from build123d import *

# Parameters (mm, degrees)
BOSS_EXTRUDE5_DEPTH      = 20
BOSS_EXTRUDE5_DEPTH_BACK = 20
SKETCH6_R                = 2.6000000000000005
SKETCH7_W                = 30.000000000000004
SKETCH7_H                = 21
CUT_EXTRUDE1_DEPTH       = 16
BOSS_EXTRUDE6_DEPTH      = 18
BOSS_EXTRUDE7_DEPTH      = 4
SKETCH12_W               = 4.9999999999999964
SKETCH12_H               = 12.999999999999998
BOSS_EXTRUDE8_DEPTH      = 34
FILLET4_R                = 5
FILLET5_R                = 1
CUT_EXTRUDE3_START       = -15
CUT_EXTRUDE3_DEPTH       = 10
CUT_EXTRUDE4_DEPTH       = 3.923095079
FILLET7_R                = 5
FILLET8_R                = 50


with BuildPart() as part:
    # Sketch6 → Boss-Extrude5 (new, two sides: drawn at the far end of the back side and taken through both)
    with BuildSketch(Plane(origin=(0, 0, 0), x_dir=(0, 0, -1), z_dir=(1, 0, 0)).offset(-BOSS_EXTRUDE5_DEPTH_BACK)):
        with BuildLine():
            Line((-23, -8), (0, -8))
            ThreePointArc((0, -8), (8, 0), (0, 8))
            Line((0, 8), (-13, 7.999999999999998))
            Line((-13, 7.999999999999998), (-13, 42))
            Line((-13, 42), (-8.56466921236316, 42))
            Line((-8.56466921236316, 42), (6.542901083469773, 68.16707933130117))
            Line((6.542901083469773, 68.16707933130117), (-5.004104300322731, 68.16707933130117))
            Line((-5.004104300322731, 68.16707933130117), (-20.111674596155662, 42))
            Line((-20.111674596155662, 42), (-23, 42))
            Line((-23, 42), (-23, -8))
        make_face()
        Circle(SKETCH6_R, mode=Mode.SUBTRACT)
    extrude(amount=BOSS_EXTRUDE5_DEPTH + BOSS_EXTRUDE5_DEPTH_BACK)

    # Sketch7 → Cut-Extrude1 (cut)
    with BuildSketch(Plane(origin=(0, 8, 1.07e-15), x_dir=(1, 0, 0), z_dir=(0, 1, 0))):
        with Locations((0, -2.4999999999999982)):
            Rectangle(SKETCH7_W, SKETCH7_H)
    extrude(amount=-CUT_EXTRUDE1_DEPTH, mode=Mode.SUBTRACT)

    # Sketch9 → Boss-Extrude6 (add)
    with BuildSketch(Plane(origin=(20, 0, 0), x_dir=(0, 0, -1), z_dir=(1, 0, 0))):
        Polygon((-8, -8), (-7.9999999999999964, -28.890618944469697), (-23, -8), align=None)
    boss_extrude6 = extrude(amount=-BOSS_EXTRUDE6_DEPTH)

    # Mirror1: Boss-Extrude6 across plane
    add(boss_extrude6.mirror(Plane(origin=(0, 0, 0), x_dir=(0, 0, 1), z_dir=(1, 0, 0))))

    # Sketch10 → Boss-Extrude7 (add)
    with BuildSketch(Plane.ZY.offset(-2)):
        Polygon((23, -8), (13, -8), (13.000000000000004, -21.927079296313124), align=None)
    extrude(amount=BOSS_EXTRUDE7_DEPTH)

    # Sketch12 → Boss-Extrude8 (add)
    with BuildSketch(Plane(origin=(0, 8, 1.07e-15), x_dir=(1, 0, 0), z_dir=(0, 1, 1.3e-16))):
        with Locations((17.5, -6.499999999999999)):
            Rectangle(SKETCH12_W, SKETCH12_H)
    boss_extrude8 = extrude(amount=BOSS_EXTRUDE8_DEPTH)

    # Mirror2: Boss-Extrude8 across plane
    add(boss_extrude8.mirror(Plane(origin=(0, 0, 0), x_dir=(0, 0, 1), z_dir=(1, 0, 0))))

    # Fillet4
    fillet4_edges = [part.edges().sort_by_distance(p)[0] for p in [
        (2, -8, 10.5),
        (-2, -8, 10.5),
    ]]
    fillet(fillet4_edges, radius=FILLET4_R)

    # Fillet5
    fillet5_edges = [part.edges().sort_by_distance(p)[0] for p in [
        (0, 68.16707933130117, -6.542901083469773),
        (11, -28.890618944469697, 7.9999999999999964),
        (-11, -28.890618944469697, 7.9999999999999964),
    ]]
    fillet(fillet5_edges, radius=FILLET5_R)

    # Sketch13 → Cut-Extrude3 (cut)
    with BuildSketch(Plane(origin=(20, 0, 0), x_dir=(0, 0, -1), z_dir=(1, 0, 0)).offset(CUT_EXTRUDE3_START)):
        Polygon((6.542901083469864, 68.16707933130117), (-8.56466921236316, 42), (-13.094669212363161, 42), (2.0129010834698517, 68.16707933130117), align=None)
    extrude(amount=-CUT_EXTRUDE3_DEPTH, mode=Mode.SUBTRACT)

    # Sketch14 → Cut-Extrude4 (cut)
    with BuildSketch(Plane(origin=(0, 14.20861055645838, 24.61003538874555), x_dir=(-1, 0, 0), z_dir=(0, -0.49999999999999784, -0.8660254037844399))):
        Polygon((-15.000000000000004, 32.090732352764924), (-5.000000000000001, 48.794944027775955), (-5.000000000000001, 32.090732352764924), (-5.000000000000001, 29.87306695894652), (-15.000000000000007, 29.87306695894652), align=None)
    cut_extrude4 = extrude(amount=-CUT_EXTRUDE4_DEPTH, mode=Mode.SUBTRACT)

    # Mirror3: Cut-Extrude4 across plane
    add(cut_extrude4.mirror(Plane(origin=(0, 0, 0), x_dir=(0, 0, 1), z_dir=(1, 0, 0))), mode=Mode.SUBTRACT)

    # Fillet7
    fillet7_edges = [part.edges().sort_by_distance(p)[0] for p in [
        (17.5, 42, 5.6e-15),
        (-17.5, 42, 5.6e-15),
        (0, 68.16707933130117, 5.004104300322731),
        (5.000000000000001, 57.44704543050219, 1.9113133747955424),
        (-5.000000000000001, 57.44704543050219, 1.9113133747955426),
    ]]
    fillet(fillet7_edges, radius=FILLET7_R)

    # Fillet8
    # the kernel refuses this fillet: 50 mm, written as the material it takes off along each edge
    with BuildSketch(Plane(origin=(61.869597916190855, 42, 23), x_dir=(0, 0, -1), z_dir=(-1, 0, 0))) as fillet8_piece_1:
        with BuildLine():
            CenterArc((50, 16.747839166469827), FILLET8_R, 180, 19.569909983271373)
            Line((0, 16.747839166469827), (-1, 16.747839166469827))
            Line((-1, 16.747839166469827), (-1, 0))
            Line((-1, 0), (0, -1))
            ThreePointArc((0, -1), (1.444162701922167, -1), (1.946091911921222, -0.33495678332939605))
            Line((1.946091911921222, -0.33495678332939605), (2.888325403844334, 0))
        make_face()
    extrude(amount=123.73919583238171, mode=Mode.SUBTRACT)
    with BuildSketch(Plane(origin=(-60.228570108654466, -8.000000000000004, 23), x_dir=(0, -0.812294131590468, -0.5832480122415225), z_dir=(1, 0, 0))) as fillet8_piece_2:
        with BuildLine():
            CenterArc((FILLET8_R * 0.321828560869, FILLET8_R), FILLET8_R, 234.32068370191269, 35.67931629808726)
            Line((-FILLET8_R * 0.261419451372, FILLET8_R * 0.18770586841), (-FILLET8_R * 0.273084411617, FILLET8_R * 0.171459985778))
            Line((-FILLET8_R * 0.273084411617, FILLET8_R * 0.171459985778), (-FILLET8_R * 0.00643657121738, -FILLET8_R * 0.02))
            Line((-FILLET8_R * 0.00643657121738, -FILLET8_R * 0.02), (FILLET8_R * 0.321828560869, -FILLET8_R * 0.02))
            Line((FILLET8_R * 0.321828560869, -FILLET8_R * 0.02), (FILLET8_R * 0.321828560869, 5e-16))
        make_face()
    extrude(amount=120.45714021730896, mode=Mode.SUBTRACT)


solid = part.part
Verification items for the finished model (mm, model axes). A direction names the side the tool comes from. Give positions to 0.01 mm unless a question says otherwise; leave off trailing zeros. Loops run counter-clockwise (first coordinate to the right, second up) from the corner with the lowest first, then second, coordinate; pieces in that order, holes last. Notation, with made-up numbers: (-7, 3) - (10, 3) arc R20 ccw to (10, 17) - close; hole circle Ø4 at (-13.75, 25.25). An arc over 180 degrees is marked (long way). Write item = value, one per line. Start each with the question number.
Q1. Depth check by flat-ended pin: P1, Ø2, axis at x = -6.5, y = 55.5, coming from the +Z side; P2, Ø2, axis at x = -4.5, y = 56.5, coming from the +Z side; P3, Ø9, axis at x = 7.5, y = -16, coming from the -Z side; P4, Ø4, axis at y = 0, z = 0, coming from the -X side. Enter the tip coordinate at first touch or a pass-through.
Q2. Cross-section at D-D, the plane y = 45. Enter the section's corners in (x, z), and give its area (3 significant figures).
Q3. Cross-section at A-A, the plane y = 0. Enter the section's corners in (x, z).
Q4. Mould release check, pull along Y, two halves, no side actions. Record for faces 4 (the face through (0.28, 67.48, 4.65)), 5 (the face through (2, -20, 10)), 6 (the face through (4, -9, 10)): released by +Y, released by -Y, zero draft, split by the parting line, or undercut.
Q5. Cross-section at B-B, the plane y = -19.5. Enter the section's corners in (x, z).
Q6. Thickness scan on line 1 (X direction, y = 38, z = 11.5); line 2 (Z direction, x = -17, y = 10.5); line 3 (X direction, y = 54.5, z = 3.5). Record the ranges inside material, lowest first.
Q7. Cross-section at C-C, the plane x = 14. Enter the section's corners in (y, z).
Q8. Tool access check on faces 1 (the face through (11, -8, 11)), 2 (the face through (11, -17, 8)), 3 (the face through (18, 40, 1)). Record the directions out of +Z, -Z, +X, -X, +Y, -Y that give a thin tool (end or side, any length) a straight path to the whole face; none if there is none.
Answer key:
q1.P1 = 12.89
q1.P2 = 12.32
q1.P3 = 8
q1.P4 = through
q2.outline = (-20, 6.83) - (-12.93, 6.83) - (-14.28, 11.36) - (14.28, 11.36) - (12.93, 6.83) - (20, 6.83) - (20, 18.38) - (-20, 18.38) - close
q2.area = 339 mm^2
q3.outline = (-20, -8) - (-15, -8) - (-15, -2.6) - (-20, -2.6) - close; (-20, 2.6) - (-15, 2.6) - (-15, 13) - (15, 13) - (15, 2.6) - (20, 2.6) - (20, 22.34) - (-20, 22.34) - close; (15, -8) - (20, -8) - (20, -2.6) - (15, -2.6) - close
q4.face_4 = released by +Y
q4.face_5 = zero draft
q4.face_6 = undercut
q5.outline = (-20, 8) - (-2, 8) - (-2, 13) - (2, 13) - (2, 8) - (20, 8) - (20, 14.7) - (-20, 14.7) - close
q6.line_1 = -20 to -15, 15 to 20
q6.line_2 = 0 to 23
q6.line_3 = -20 to -7, 7 to 20
q7.outline = (-26.37, 9.81) arc R1 ccw to (-25.78, 8) - (-8, 8) - (-8, 13) - (42, 13) - (42.04, 13.07) - (45.41, 11.13) - (43.45, 7.73) - (66.67, -5.68) arc R1 ccw to (68.17, -4.81) - (68.17, 2.12) arc R5 ccw to (65.67, 6.45) - (42, 20.11) arc R50 ccw to (25.25, 23) - (8.09, 23) arc R50 ccw to (-21.07, 13.61) - close
q8.face_1 = -Z
q8.face_2 = -Z, +X, -X, -Y
q8.face_3 = -Z, +X, -X
